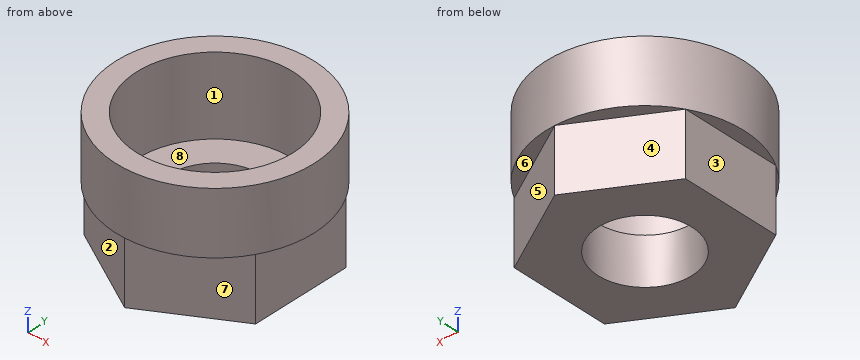
from build123d import *

# Parameters (mm, degrees)
SKETCH_R        = 9.5
PAD_DEPTH       = 6
PAD001_DEPTH    = 6
SKETCH002_R     = 4.5
POCKET_DEPTH    = 8
SKETCH003_R     = 7.5
POCKET001_DEPTH = 7.5


with BuildPart() as part:
    # Sketch → Pad (new body)
    with BuildSketch(Plane.XY):
        Circle(SKETCH_R)
    extrude(amount=-PAD_DEPTH)

    # Sketch001 → Pad001 (new body)
    with BuildSketch(Plane(origin=(0, 0, -6), x_dir=(1, 0, 0), z_dir=(0, 0, -1))):
        Polygon((8.227241, -4.75), (8.227241, 4.75), (0, 9.5), (-8.227241, 4.75), (-8.227241, -4.75), (0, -9.5), align=None)
    extrude(amount=PAD001_DEPTH)

    # Sketch002 → Pocket (cut)
    with BuildSketch(Plane(origin=(0, 0, -12), x_dir=(1, 0, 0), z_dir=(0, 0, -1))):
        Circle(SKETCH002_R)
    extrude(amount=-POCKET_DEPTH, mode=Mode.SUBTRACT)

    # Sketch003 → Pocket001 (cut)
    with BuildSketch(Plane.XY):
        Circle(SKETCH003_R)
    extrude(amount=-POCKET001_DEPTH, mode=Mode.SUBTRACT)


solid = part.part
Geometry check sheet. Reference: the model listing, model coordinates, mm. Face numbers are marked on the shaded views. A direction names the side the tool comes from. Round coordinates to 2 decimals unless told otherwise and drop trailing zeros. Order: outer loops, then holes, each group sorted by start corner. A loop starts at its lowest first (then second) coordinate and runs counter-clockwise, first axis right, second up. Notation, with made-up numbers: (-14, -5) - (5, -5) arc R24 ccw to (5, 22) - close; hole circle Ø7 at (-13.5, -19). An arc over 180 degrees is marked (long way). One line per question, with ' | ' between items. Start each with the question number.
(1) Thickness scan on L1, parallel to X at y = 0, z = -10; L2, parallel to Y at x = 0, z = -3.5; L3, parallel to Z at x = 7, y = -5.5. Record the ranges inside material, lowest first. Write a range as [from, to].
(2) Sectioned sample at C-C on z = -4.5. Record the cut outline in (x, y), and give its area (3 significant figures).
(3) Release check for a two-part mould opening along Y. For the marked faces 6, 7 and 8 record: released by +Y, released by -Y, zero draft, split by the parting line, or undercut.
(4) Depth check by flat-ended pin: pin 1 Ø1 at (y, z) = (-5.5, -7.5) entering from +X; pin 2 Ø1.4 at (x, y) = (5.5, 7.5) entering from -Z; pin 3 Ø3 at (y, z) = (-2, -8) entering from -X. Enter the tip coordinate at first touch or a pass-through.
(5) Sectioned sample at D-D on x = 6.5. Record the cut outline in (y, z), and give its area (3 significant figures).
(6) Sectioned sample at B-B on x = -4.25. Record the cut outline in (y, z).
(7) Sectioned sample at A-A on y = 0. Record the cut outline in (x, z).
(8) Access from +Z, -Z, +X, -X, +Y, -Y to the whole of each face (thin tool, end or side, straight path). Record for the marked faces 1, 2, 3, 4 and 5.
Conclusion:
1) L1: x = [-8.23, -4.5], [4.5, 8.23] | L2: y = [-9.5, -7.5], [7.5, 9.5] | L3: z = [-6, 0]
2) outline: circle Ø19 at (0, 0); hole circle Ø15 at (0, 0) | area: 107 mm2
3) face 6: zero draft | face 7: released by -Y | face 8: undercut
4) pin 1: stops at x = 7.79 | pin 2: stops at z = -6 | pin 3: stops at x = -8.23
5) outline: (-6.93, -6) - (-5.75, -6) - (-5.75, -12) - (5.75, -12) - (5.75, -6) - (6.93, -6) - (6.93, 0) - (3.74, 0) - (3.74, -7.5) - (-3.74, -7.5) - (-3.74, 0) - (-6.93, 0) - close | area: 96.0 mm2
6) outline: (-8.5, -6) - (-7.05, -6) - (-7.05, -12) - (-1.48, -12) - (-1.48, -7.5) - (-6.18, -7.5) - (-6.18, 0) - (-8.5, 0) - close; (1.48, -12) - (7.05, -12) - (7.05, -6) - (8.5, -6) - (8.5, 0) - (6.18, 0) - (6.18, -7.5) - (1.48, -7.5) - close
7) outline: (-9.5, -6) - (-8.23, -6) - (-8.23, -12) - (-4.5, -12) - (-4.5, -7.5) - (-7.5, -7.5) - (-7.5, 0) - (-9.5, 0) - close; (4.5, -12) - (8.23, -12) - (8.23, -6) - (9.5, -6) - (9.5, 0) - (7.5, 0) - (7.5, -7.5) - (4.5, -7.5) - close
8) face 1: +Z | face 2: -Z, -X, -Y | face 3: -Z, -X, +Y, -Y | face 4: -Z, -X, +Y | face 5: -Z, +X, +Y
